```python
from build123d import *

# Parameters (mm, degrees)
BOSS_EXTRUDE1_DEPTH      = 1000
BOSS_EXTRUDE1_DEPTH_BACK = 1000


with BuildPart() as part:
    # Sketch1 → Boss-Extrude1 (new body, two sides)
    with BuildSketch(Plane.XY) as boss_extrude1_sk:
        with BuildLine():
            Line((-14, -16), (14, -16))
            ThreePointArc((14, -16), (15.414213562, -15.414213562), (16, -14))
            Line((16, -14), (16, 14))
            ThreePointArc((16, 14), (15.414213562, 15.414213562), (14, 16))
            Line((14, 16), (-14, 16))
            ThreePointArc((-14, 16), (-15.414213562, 15.414213562), (-16, 14))
            Line((-16, 14), (-16, -14))
            ThreePointArc((-16, -14), (-15.414213562, -15.414213562), (-14, -16))
        make_face()
        with BuildLine():
            Line((-14, 14.48), (14, 14.48))
            ThreePointArc((14, 14.48), (14.339411255, 14.339411255), (14.48, 14))
            Line((14.48, 14), (14.48, -14))
            ThreePointArc((14.48, -14), (14.339411255, -14.339411255), (14, -14.48))
            Line((14, -14.48), (-14, -14.48))
            ThreePointArc((-14, -14.48), (-14.339411255, -14.339411255), (-14.48, -14))
            Line((-14.48, -14), (-14.48, 14))
            ThreePointArc((-14.48, 14), (-14.339411255, 14.339411255), (-14, 14.48))
        make_face(mode=Mode.SUBTRACT)
    extrude(amount=BOSS_EXTRUDE1_DEPTH)
    extrude(boss_extrude1_sk.sketch, amount=-BOSS_EXTRUDE1_DEPTH_BACK)


solid = part.part
```
The model under review builds one solid part; all positions refer to its coordinate system, in mm. Round coordinates to 2 decimals unless told otherwise and drop trailing zeros. Write each loop counter-clockwise with the first axis right and the second up, starting at its lowest first coordinate (ties: lowest second). Pieces come first, ordered by that corner, then holes.
(1) Wall thickness on L1, parallel to X at y = 6, z = 569; L2, parallel to Y at x = -15, z = 721: over which ranges is each line inside the solid? List them lowest first.
(2) We need section A-A on y = -7.5. Give the boundary of the cut face in (x, z), and give its area (3 significant figures).
(3) We need section B-B on z = -621. Give the boundary of the cut face in (x, y).
Findings below:
1. L1: x = -16 to -14.48, 14.48 to 16
1. L2: y = -15.73 to 15.73
2. outline: (-16, -1000) - (-14.48, -1000) - (-14.48, 1000) - (-16, 1000) - close; (14.48, -1000) - (16, -1000) - (16, 1000) - (14.48, 1000) - close
2. area: 6,080 mm2
3. outline: (-16, -14) arc R2 ccw to (-14, -16) - (14, -16) arc R2 ccw to (16, -14) - (16, 14) arc R2 ccw to (14, 16) - (-14, 16) arc R2 ccw to (-16, 14) - close; hole (-14.48, -14) arc R0.48 ccw to (-14, -14.48) - (14, -14.48) arc R0.48 ccw to (14.48, -14) - (14.48, 14) arc R0.48 ccw to (14, 14.48) - (-14, 14.48) arc R0.48 ccw to (-14.48, 14) - close
